Could you check a few things on this drawing? It's one solid part, dimensions in mm from its lowest x, y, z. A direction names the side the tool comes from. Coordinates: 2 decimals unless noted, no trailing zeros. Loops run counter-clockwise (first coordinate to the right, second up) from the corner with the lowest first, then second, coordinate; pieces in that order, holes last. Notation, with made-up numbers: M -22.75,69 L 8.25,69 A14 cw 8.25,80 Z; hole C 24,53.25 d6. An arc over 180 degrees is marked long. Answer as a JSON object with one key per item and string values. Group by question number.
Item 1: Suppose I cut it at D-D (z = 17.75). Write out the boundary of the cut face in (x, y).
Item 2: We'd pull the mould along X, two halves only. Please class the marked faces 3, 4 and 5: +X half, -X half, draft (parallel to the pull), parting line (faces both ways), or undercut.
Item 3: Suppose I cut it at A-A (z = 10). Write out the boundary of the cut face in (x, y).
Item 4: Which directions (+Z, -Z, +X, -X, +Y, -Y) give clear straight access to the entire face, cutting with the end or side of a thin tool? Please do the marked faces 1 and 2.
Item 5: Suppose I cut it at B-B (x = 14). Write out the boundary of the cut face in (y, z).
Item 6: If I drill on line 1 (X direction, y = 7.5, z = 10); line 2 (X direction, y = 16, z = 17.75); line 3 (Z direction, x = 71, y = 11.25), over which ranges is the centre line in solid material (lowest first)?
Item 7: Suppose I cut it at C-C (y = 8). Write out the boundary of the cut face in (x, z).
Item 8: I'm going to push flat-ended pins straight in: pin 1 Ø5 at (x, z) = (90, 17) entering from -Y; pin 2 Ø1 at (x, z) = (79, 5) entering from +Y; pin 3 Ø8 at (x, z) = (12.5, 4) entering from +Y. Where does each tip first touch, or does it pass through?
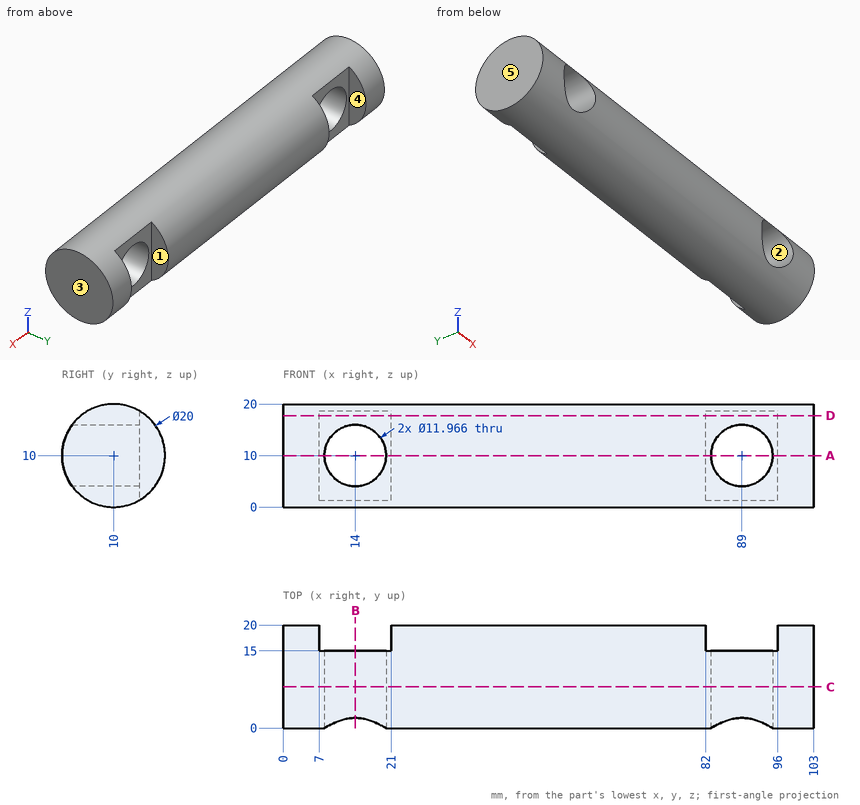
From the geometry:
{
 "1": {"outline": "M 0,3.68 L 103,3.68 L 103,16.32 L 96,16.32 L 96,15 L 82,15 L 82,16.32 L 21,16.32 L 21,15 L 7,15 L 7,16.32 L 0,16.32 Z"},
 "2": {"face 3": "+X half", "face 4": "undercut", "face 5": "-X half"},
 "3": {"outline": "M 0,0 L 8.02,0 L 8.02,15 L 7,15 L 7,20 L 0,20 Z; M 19.98,0 L 83.02,0 L 83.02,15 L 82,15 L 82,20 L 21,20 L 21,15 L 19.98,15 Z; M 94.98,0 L 103,0 L 103,20 L 96,20 L 96,15 L 94.98,15 Z"},
 "4": {"face 1": "+Z, -Z, +Y", "face 2": "+Y, -Y"},
 "5": {"outline": "M 1.99,4.02 A10 ccw 15,1.34 L 15,4.02 Z; M 1.99,15.98 L 15,15.98 L 15,18.66 A10 ccw Z"},
 "6": {"line 1": "0 to 8.02, 19.98 to 83.02, 94.98 to 103", "line 2": "0 to 7, 21 to 82, 96 to 103", "line 3": "0.08 to 19.92"},
 "7": {"outline": "M 0,0.2 L 103,0.2 L 103,19.8 L 0,19.8 Z; hole C 14,10 d11.97; hole C 89,10 d11.97"},
 "8": {"pin 1": "y = 1.51", "pin 2": "y = 18.93", "pin 3": "y = 15"}
}
